Part model, mm, in its own coordinate system. A direction names the side the tool comes from. Coordinates: 2 decimals unless noted, no trailing zeros. Loops run counter-clockwise (first coordinate to the right, second up) from the corner with the lowest first, then second, coordinate; pieces in that order, holes last. Notation, with made-up numbers: (-13.5, 89.5) - (37.5, 89.5) arc R29 cw to (37.5, 115.5) - close; hole circle Ø4 at (-17, 46). An arc over 180 degrees is marked (long way). One line per question, with ' | ' between items. Start each with the question number.
from build123d import *

# Parameters (mm, degrees)
F0_W       = 38.1
F0_H       = 38.1
F1_ANGLE   = 68.5
F3_DEPTH   = 38.101
F1_FACE1_W = 38.1
F1_FACE1_H = 38.1
F4_ANGLE   = 22
F5_R       = 1.4986
F6_R       = 1.4986
F7_DEPTH   = 6.35
F8_R       = 1.4986
F9_DEPTH   = 6.35


with BuildPart() as f1:
    # F0 (on Top) → F1 (revolve)
    with BuildSketch(Plane.XY):
        with Locations((0.4687455922, 2.6705784231)):
            Rectangle(F0_W, F0_H)
    revolve(axis=Axis((0.4687455922, -16.3794215769, 0), (1, 0, 0)), revolution_arc=F1_ANGLE)

    # F2 (on face) → F3 (cut, through all)
    with BuildSketch(Plane(origin=(-18.5812544078, 0, 0), x_dir=(0, -1, 0), z_dir=(-1, 0, 0))):
        with BuildLine():
            Line((-21.7205784231, 0), (2.4157248387, 35.4489093401))
            ThreePointArc((2.4157248387, 35.4489093401), (-15.1136478649, 21.4428677452), (-21.7205784231, 0))
        make_face()
    extrude(amount=-F3_DEPTH, mode=Mode.SUBTRACT)

    # F1_face1 (on face) → F4 (revolve)
    with BuildSketch(Plane(origin=(0.4687455922, -9.3975732078, 17.7244546701), x_dir=(1, 0, 0), z_dir=(0, -0.930417568, 0.3665012267))):
        Rectangle(F1_FACE1_W, F1_FACE1_H)
    revolve(axis=Axis((0.4687455922, -16.3794215769, 0), (1, 0, 0)), revolution_arc=F4_ANGLE)

    # F5 (on face) + F6 (on face) → F7 (cut)
    with BuildSketch(Plane(origin=(0, -16.3781742442, -0.1429301613), x_dir=(1, 0, 0), z_dir=(0, -0.9999619231, -0.0087265355))):
        with Locations((-7.6464321464, 19.1929356038)):
            Circle(F5_R)
    with BuildSketch(Plane(origin=(0, -16.3781742442, -0.1429301613), x_dir=(1, 0, 0), z_dir=(0, -0.9999619231, -0.0087265355))):
        with Locations((8.3530278536, 19.1929356038)):
            Circle(F6_R)
    extrude(amount=-F7_DEPTH, mode=Mode.SUBTRACT)

    # F8 (on face) → F9 (cut)
    with BuildSketch(Plane(origin=(0, 14.8405985302, 10.1046038758), x_dir=(-1, 0, 0), z_dir=(0, 0.8265897491, 0.5628049277))):
        with Locations((-9.9312769204, 8.9093865827)):
            Circle(F8_R)
        with Locations((6.0707230796, 8.9093865827)):
            Circle(F8_R)
    extrude(amount=-F9_DEPTH, mode=Mode.SUBTRACT)


solid = f1.part
1) Pin check, flat tips, straight feed: pin 1 Ø1 at (x, z) = (11.5, 13.5) entering from +Y; pin 2 Ø10 at (x, y) = (11.5, 12.5) entering from +Z; pin 3 Ø12 at (x, z) = (4.5, 21.5) entering from -Y. Stop position of each tip, or through.
2) Band-saw the part on B-B on z = 25. List the corners of the cut face in (x, y).
3) Mould opens along Y. For faces 1 (the flat face through (0.2, 9.82, 17.48)), 2 (the cylindrical face through (-4.574, 7.202, 15.762)), 3 (the flat face through (-18.581, 0, 14)) say: +Y half, -Y half, draft (parallel to the pull), parting line (faces both ways), or undercut.
4) Band-saw the part on C-C on y = -12. Count the separate pieces of the cut face and the enclosed holes in it, then the cut area to 3 significant figures.
5) Tool access for faces 4 (the flat face through (0, 3, 0)), 5 (the cylindrical face through (7.25, -13.42, 20.09)): list every direction of +Z, -Z, +X, -X, +Y, -Y with a clear straight run to the whole face (end or side of a thin tool).
6) Band-saw the part on A-A on x = -11. List the corners of the cut face in (y, z).
7) Wall check: line 1 along Z through (x, y) = (9, 9); line 2 along Z through (x, y) = (14.5, 16); line 3 along Z through (x, y) = (18, 5.5). Give the ranges that are in metal, low to high. Write a range as [from, to].
Values found:
1) pin 1: y = 12.87 | pin 2: z = 20.89 | pin 3: y = -16.62
2) outline: (-18.58, -16.6) - (19.52, -16.6) - (19.52, 4.7) - (-18.58, 4.7) - close
3) face 1: +Y half | face 2: undercut | face 3: draft
4) separate pieces: 1 | enclosed holes: 2 | area: 1,430 mm²
5) face 4: -Z, +X, -X, +Y, -Y | face 5: none
6) outline: (-16.71, 38.1) - (-16.38, 0) - (21.72, 0) - (-2.42, 35.45) arc R38.1 ccw to start
7) line 1: [0, 15.49], [18.33, 18.68] | line 2: [0, 8.4] | line 3: [0, 23.82]
